Could you check a few things on this drawing? It's one solid part, dimensions in mm from its lowest x, y, z. A direction names the side the tool comes from. Round coordinates to 2 decimals unless told otherwise and drop trailing zeros. Write each loop counter-clockwise with the first axis right and the second up, starting at its lowest first coordinate (ties: lowest second). Pieces come first, ordered by that corner, then holes. Notation, with made-up numbers: M 55,53 L 102,53 A19 ccw 102,77 Z; hole C 35,-36 d5. An arc over 180 degrees is marked long. One line per item, written item: value. Start each with the question number.
(1) I want a section at A-A on x = 10. Please give me the cut outline in (y, z).
(2) Thinking about a two-plate mould opening in Z: for the marked faces 5, 6 and 7, which applies, released by +Z, released by -Z, zero draft, split by the parting line, or undercut?
(3) Which directions (+Z, -Z, +X, -X, +Y, -Y) give clear straight access to the entire face, cutting with the end or side of a thin tool? Please do the marked faces 1, 2, 3 and 4.
(4) I want a section at C-C on z = 13.5. Please give me the cut outline in (x, y).
(5) I want a section at B-B on y = 10. Please give me the cut outline in (x, z).
(6) I'm going to push flat-ended pins straight in: pin 1 Ø8 at (x, y) = (16.5, 12) entering from -Z; pin 2 Ø1.5 at (y, z) = (5, 10) entering from -X (1 decimal); pin 3 Ø10 at (y, z) = (4, 4.5) entering from +X; pin 4 Ø1 at (y, z) = (12.5, 13.5) entering from -X. Where does each tip first touch, or does it pass through?
(7) If I drill on L1, parallel to Y at x = 10, z = 14.3; L2, parallel to Y at x = 10, z = 16.75; L3, parallel to Z at x = 5, y = 4.5, over which ranges is the centre line in solid material (lowest first)?
(8) I want a section at D-D on z = 2.5. Please give me the cut outline in (x, y), and give its area (3 significant figures).
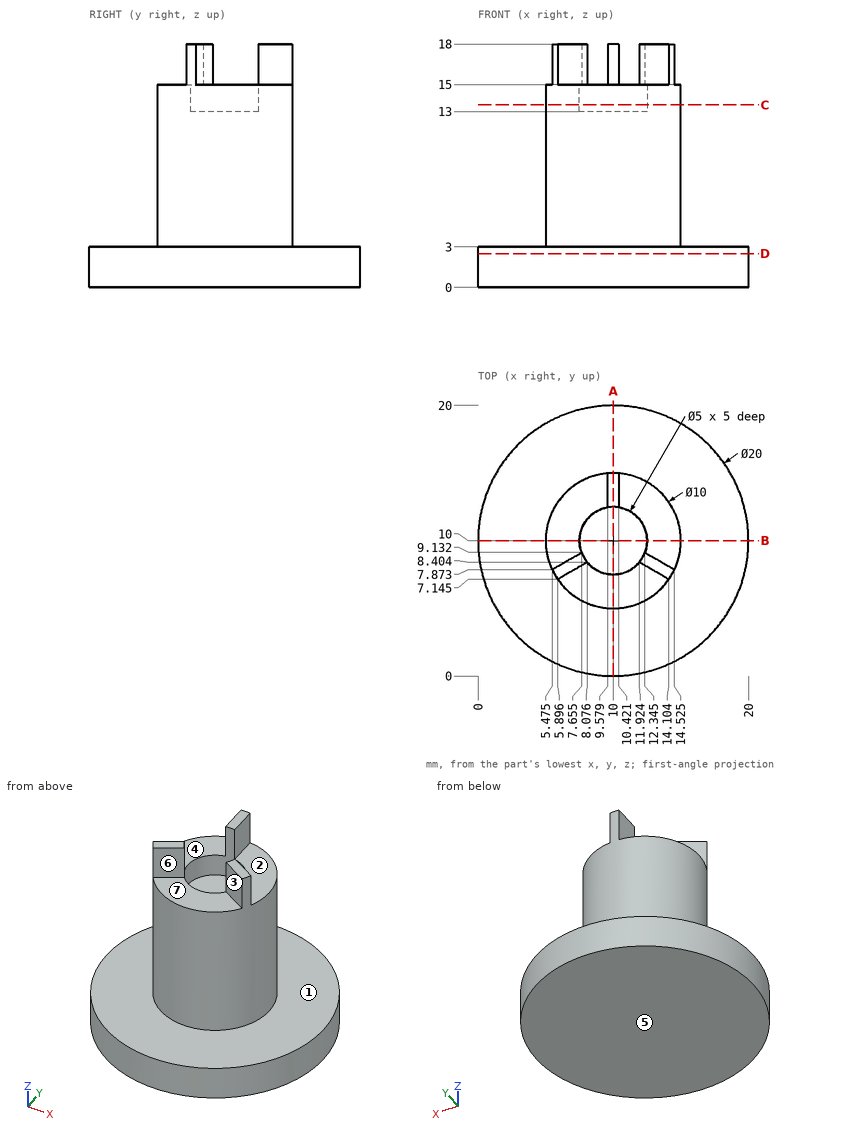
Found:
1. outline: M 0,0 L 20,0 L 20,3 L 15,3 L 15,18 L 12.5,18 L 12.5,13 L 7.5,13 L 7.5,15 L 5,15 L 5,3 L 0,3 Z
2. face 5: released by -Z
2. face 6: zero draft
2. face 7: released by +Z
3. face 1: +Z
3. face 2: +Z, +X, +Y
3. face 3: +Z, -Y
3. face 4: +Z, -X, +Y
4. outline: C 10,10 d10; hole C 10,10 d5
5. outline: M 0,0 L 20,0 L 20,3 L 15,3 L 15,15 L 12.5,15 L 12.5,13 L 7.5,13 L 7.5,15 L 5,15 L 5,3 L 0,3 Z
6. pin 1: stops at z = 0
6. pin 2: stops at x = 7.4
6. pin 3: stops at x = 19.92
6. pin 4: stops at x = 5.42
7. L1: y = 5 to 7.5, 12.5 to 15
7. L2: y = 12.5 to 15
7. L3: z = 0 to 3
8. outline: C 10,10 d20
8. area: 314 mm²
